from build123d import *

# Parameters (mm, degrees)
SKETCH_1_W      = 165
SKETCH_1_H      = 64
SKETCH_1_R      = 2
SKETCH_1_R_2    = 2.15
SKETCH_1_R_3    = 11
EXTRUDE_1_DEPTH = 4
FILLET_1_R      = 10


with BuildPart() as part:
    # 草图1 → 凸台-拉伸1 (new body)
    with BuildSketch(Plane(origin=(0, 0, 0), x_dir=(1, 0, 0), z_dir=(0, 1, 0))):
        with Locations((82.5, 32)):
            Rectangle(SKETCH_1_W, SKETCH_1_H)
        with Locations(Location((10, 57, 0), (0, 0, 270))):
            Circle(SKETCH_1_R, mode=Mode.SUBTRACT)
        with Locations(Location((155, 57, 0), (0, 0, 270))):
            Circle(SKETCH_1_R, mode=Mode.SUBTRACT)
        with Locations(Location((155, 7, 0), (0, 0, 270))):
            Circle(SKETCH_1_R, mode=Mode.SUBTRACT)
        with Locations(Location((10, 7, 0), (0, 0, 270))):
            Circle(SKETCH_1_R, mode=Mode.SUBTRACT)
        with Locations(Location((102.5, 47.5, 0), (0, 0, 270))):
            Circle(SKETCH_1_R_2, mode=Mode.SUBTRACT)
        with Locations(Location((87, 32, 0), (0, 0, 270))):
            Circle(SKETCH_1_R_2, mode=Mode.SUBTRACT)
        with Locations(Location((102.5, 16.5, 0), (0, 0, 270))):
            Circle(SKETCH_1_R_2, mode=Mode.SUBTRACT)
        with Locations(Location((118, 32, 0), (0, 0, 270))):
            Circle(SKETCH_1_R_2, mode=Mode.SUBTRACT)
        with Locations(Location((102.5, 32, 0), (0, 0, 270))):
            Circle(SKETCH_1_R_3, mode=Mode.SUBTRACT)
    extrude(amount=EXTRUDE_1_DEPTH)

    # 圆角1
    fillet_1_edges = [part.edges().sort_by_distance(p)[0] for p in [
        (0, 2, -64),
        (165, 2, -64),
        (165, 2, 0),
        (0, 2, 0),
    ]]
    fillet(fillet_1_edges, radius=FILLET_1_R)


solid = part.part
The listing builds one solid part. Answer for the finished solid, in the listing's coordinates (mm). Give positions to 0.01 mm unless a question says otherwise; leave off trailing zeros. Loops run counter-clockwise (first coordinate to the right, second up) from the corner with the lowest first, then second, coordinate; pieces in that order, holes last. Notation, with made-up numbers: (66.25, 43.25) - (77.25, 43.25) arc R18 cw to (77.25, 59.25) - close; hole circle Ø11 at (47, -24). An arc over 180 degrees is marked (long way). Answer as a JSON object with one key per item and string values.
1. For a pull along Z with two mould halves and no side action, classify faces 1 (the cylindrical face through (161.99, 2.03, -2.85)), 2 (the flat face through (81, 2, -64)), 3 (the cylindrical face through (11.352, 1.972, -8.474)) as pulls with the +Z half, pulls with the -Z half, needs draft (parallel to the pull), parting line crosses it, or undercut.
Determined:
{"face 1": "pulls with the +Z half", "face 2": "pulls with the -Z half", "face 3": "undercut"}
2. A cutting plane is placed at B-B (y = 2.75). Give the number of separate pieces and of enclosed holes in the cut face, then the cut area to 3 significant figures.
Determined:
{"separate pieces": "1", "enclosed holes": "9", "area": "9,990 mm²"}
3. A cutting plane is placed at C-C (x = 102.5). Write down the section's boundary in (y, z), then the cut area to 3 significant figures.
Determined:
{"outline": "(0, -64) - (4, -64) - (4, -49.65) - (0, -49.65) - close; (0, -45.35) - (4, -45.35) - (4, -43) - (0, -43) - close; (0, -21) - (4, -21) - (4, -18.65) - (0, -18.65) - close; (0, -14.35) - (4, -14.35) - (4, 0) - (0, 0) - close", "area": "134 mm²"}
4. A cutting plane is placed at D-D (z = -47.5). Write down the section's boundary in (x, y), then the cut area to 3 significant figures.
Determined:
{"outline": "(0, 0) - (100.35, 0) - (100.35, 4) - (0, 4) - close; (104.65, 0) - (165, 0) - (165, 4) - (104.65, 4) - close", "area": "643 mm²"}
5. Find the intervals of material crossed by L1, parallel to X at y = 2.9, z = -32; L2, parallel to Z at x = 155, y = 2.05; L3, parallel to X at y = 2.95, z = -7, in increasing order. Write a range as [from, to].
Determined:
{"L1": "[0, 84.85], [89.15, 91.5], [113.5, 115.85], [120.15, 165]", "L2": "[-64, -59], [-55, -9], [-5, 0]", "L3": "[0.46, 8], [12, 153], [157, 164.54]"}
6. A cutting plane is placed at A-A (z = -32). Write down the section's boundary in (x, y).
Determined:
{"outline": "(0, 0) - (84.85, 0) - (84.85, 4) - (0, 4) - close; (89.15, 0) - (91.5, 0) - (91.5, 4) - (89.15, 4) - close; (113.5, 0) - (115.85, 0) - (115.85, 4) - (113.5, 4) - close; (120.15, 0) - (165, 0) - (165, 4) - (120.15, 4) - close"}
